from build123d import *

# Parameters (mm, degrees)
SKETCH1_W                      = 660
SKETCH1_H                      = 165
BASE_FLANGE1_DEPTH             = 1
EDGE_FLANGE1_STRIP_W           = 6
EDGE_FLANGE1_STRIP_H           = 1
EDGE_FLANGE1_STRIP_CUT_DEPTH   = 165
EDGE_FLANGE1_STRIP_2_W         = 6
EDGE_FLANGE1_STRIP_2_H         = 1
EDGE_FLANGE1_STRIP_CUT_2_DEPTH = 165
EDGE_FLANGE1_DEPTH             = 165
EDGE_FLANGE1_BEND_DEPTH        = 165
SKETCH12_W                     = 80
SKETCH12_H                     = 30
CUT_EXTRUDE1_DEPTH             = 853.027141586


# Sheet-metal steps are written as plain solids
with BuildPart() as part:
    # Sketch1 → Base-Flange1 (new body)
    with BuildSketch(Plane.XY):
        Rectangle(SKETCH1_W, SKETCH1_H)
    extrude(amount=-BASE_FLANGE1_DEPTH)

    # Edge-Flange1 strip (across the edge) → Edge-Flange1 strip cut (cut)
    with BuildSketch(Plane(origin=(330, 82.5, -1), x_dir=(-1, 0, 0), z_dir=(0, -1, 0))):
        with Locations((-2, -0.5)):
            Rectangle(EDGE_FLANGE1_STRIP_W, EDGE_FLANGE1_STRIP_H)
    extrude(amount=EDGE_FLANGE1_STRIP_CUT_DEPTH, mode=Mode.SUBTRACT)

    # Edge-Flange1 strip 2 (across the edge) → Edge-Flange1 strip cut 2 (cut)
    with BuildSketch(Plane(origin=(-330, -82.5, -1), x_dir=(1, 0, 0), z_dir=(0, 1, 0))):
        with Locations((-2, -0.5)):
            Rectangle(EDGE_FLANGE1_STRIP_2_W, EDGE_FLANGE1_STRIP_2_H)
    extrude(amount=EDGE_FLANGE1_STRIP_CUT_2_DEPTH, mode=Mode.SUBTRACT)

    # Edge-Flange1 section (across the edge) → Edge-Flange1 (add)
    with BuildSketch(Plane(origin=(330, 82.5, -1), x_dir=(-1, 0, 0), z_dir=(0, -1, 0))):
        with BuildLine():
            Line((-1, 1), (-1, 529))
            Line((-1, 529), (0, 529))
            Line((0, 529), (0, 1))
            ThreePointArc((0, 1), (0.292893219, 0.292893219), (1, 0))
            Line((1, 0), (1, -1))
            ThreePointArc((1, -1), (-0.414213562, -0.414213562), (-1, 1))
        make_face()
    extrude(amount=EDGE_FLANGE1_DEPTH)

    # Edge-Flange1 section 2 (across the edge) → Edge-Flange1 bend (add)
    with BuildSketch(Plane(origin=(-330, -82.5, -1), x_dir=(1, 0, 0), z_dir=(0, 1, 0))):
        with BuildLine():
            Line((-1, 1), (-1, 529))
            Line((-1, 529), (0, 529))
            Line((0, 529), (0, 1))
            ThreePointArc((0, 1), (0.292893219, 0.292893219), (1, 0))
            Line((1, 0), (1, -1))
            ThreePointArc((1, -1), (-0.414213562, -0.414213562), (-1, 1))
        make_face()
    extrude(amount=EDGE_FLANGE1_BEND_DEPTH)

    # Sketch12 → Cut-Extrude1 (cut, through all)
    with BuildSketch(Plane(origin=(331, 0, 0), x_dir=(0, 0, -1), z_dir=(1, 0, 0))):
        with Locations((490, 67.5)):
            Rectangle(SKETCH12_W, SKETCH12_H)
    extrude(amount=-CUT_EXTRUDE1_DEPTH, mode=Mode.SUBTRACT)


solid = part.part
Source: CAD feature listing. Evaluate the final solid. Frame: model axes, mm. Coordinates: 2 decimals unless noted, no trailing zeros. Order: outer loops, then holes, each group sorted by start corner. A loop starts at its lowest first (then second) coordinate and runs counter-clockwise, first axis right, second up.
Item 1: Cut plane C-C (z = -112.5). Return loops of the section in (x, y), plus the area to 3 significant figures.
Output values:
outline: (-331, -82.5) - (-330, -82.5) - (-330, 82.5) - (-331, 82.5) - close; (330, -82.5) - (331, -82.5) - (331, 82.5) - (330, 82.5) - close
area: 330 mm2
Item 2: Material intervals for line 1 (X direction, y = 11, z = -326.5); line 2 (Z direction, x = -210.5, y = 7), sorted ascending.
Output values:
line 1: x = -331 to -330, 330 to 331
line 2: z = -1 to 0
Item 3: First-contact query: P1, Ø8, axis at x = -34, y = -24, coming from the -Z side; P2, Ø0.5, axis at x = 330.5, z = -498, coming from the +Y side; P3, Ø3, axis at x = 212, y = 41, coming from the +Z side; P4, Ø1.1, axis at x = 330.5, y = 64.5, coming from the -Z side. Flat tips, straight axial feed; report the tip coordinate or a pass-through.
Output values:
P1: stops at z = -1
P2: stops at y = 52.5
P3: stops at z = 0
P4: stops at z = -450
Item 4: Cut plane A-A (z = -459). Return loops of the section in (x, y), plus the area to 3 significant figures.
Output values:
outline: (-331, -82.5) - (-330, -82.5) - (-330, 52.5) - (-331, 52.5) - close; (330, -82.5) - (331, -82.5) - (331, 52.5) - (330, 52.5) - close
area: 270 mm2
Item 5: Pull-direction query (X, two-part tool) for faces 1 (the face through (-5, 1, -1)), 2 (the face through (-331, -1, -262)), 3 (the face through (331, 1, -262)), 4 (the face through (-5, 1, 0)); classes: pulls with the +X half, pulls with the -X half, needs draft (parallel to the pull), parting line crosses it, or undercut.
Output values:
face 1: undercut
face 2: pulls with the -X half
face 3: pulls with the +X half
face 4: needs draft
Item 6: Cut plane B-B (y = -66). Return loops of the section in (x, z), plus the area to 3 significant figures.
Output values:
outline: (-331, -530) - (-330, -530) - (-330, -2) arc R1 cw to (-329, -1) - (329, -1) arc R1 cw to (330, -2) - (330, -530) - (331, -530) - (331, -2) arc R2 ccw to (329, 0) - (-329, 0) arc R2 ccw to (-331, -2) - close
area: 1,720 mm2
Item 7: Cut plane D-D (y = 71.5). Return loops of the section in (x, z).
Output values:
outline: (-331, -450) - (-330, -450) - (-330, -2) arc R1 cw to (-329, -1) - (329, -1) arc R1 cw to (330, -2) - (330, -450) - (331, -450) - (331, -2) arc R2 ccw to (329, 0) - (-329, 0) arc R2 ccw to (-331, -2) - close
